```python
from build123d import *

# Parameters (mm, degrees)
SKETCH1_R               = 19.05
BOSS_EXTRUDE1_DEPTH     = 5.08
SKETCH4_R               = 9.398
BOSS_EXTRUDE2_DEPTH     = 7.112
SKETCH5_R               = 2.921
CUT_EXTRUDE1_DEPTH      = 28.863695807
CUT_EXTRUDE1_DEPTH_BACK = 3.429
SKETCH6_R               = 1.4605
SKETCH6_R_2             = 1.73706236
CUT_EXTRUDE2_DEPTH      = 28.863695807
CUT_EXTRUDE2_DEPTH_BACK = 28.863695807
CUT_EXTRUDE5_DEPTH      = 3.175
SKETCH10_R              = 1.5875
CUT_EXTRUDE6_DEPTH      = 7.62


with BuildPart() as part:
    # Sketch1 → Boss-Extrude1 (new body)
    with BuildSketch(Plane(origin=(0, 0, 0), x_dir=(1, 0, 0), z_dir=(0, 1, 0))):
        with Locations(Location((0, 0, 0), (0, 0, 270))):
            Circle(SKETCH1_R)
    extrude(amount=BOSS_EXTRUDE1_DEPTH)

    # Sketch4 → Boss-Extrude2 (add)
    with BuildSketch(Plane(origin=(0, 5.08, 0), x_dir=(1, 0, 0), z_dir=(0, 1, 0))):
        with Locations(Location((0, 0, 0), (0, 0, 270))):
            Circle(SKETCH4_R)
    extrude(amount=BOSS_EXTRUDE2_DEPTH)

    # Sketch5 → Cut-Extrude1 (cut, two sides)
    with BuildSketch(Plane(origin=(0, 5.08, 0), x_dir=(1, 0, 0), z_dir=(0, 1, 0))) as cut_extrude1_sk:
        with Locations(Location((-11.43, 0, 0), (0, 0, 40.395058429))):
            Circle(SKETCH5_R)
        with Locations(Location((11.43, 0, 0), (0, 0, 139.604941571))):
            Circle(SKETCH5_R)
    extrude(amount=CUT_EXTRUDE1_DEPTH, mode=Mode.SUBTRACT)
    extrude(cut_extrude1_sk.sketch, amount=-CUT_EXTRUDE1_DEPTH_BACK, mode=Mode.SUBTRACT)

    # Sketch6 → Cut-Extrude2 (cut, two sides)
    with BuildSketch(Plane(origin=(0, 5.08, 0), x_dir=(1, 0, 0), z_dir=(0, 1, 0))) as cut_extrude2_sk:
        with Locations(Location((-11.43, 0, 0), (0, 0, 270))):
            Circle(SKETCH6_R)
        with Locations(Location((11.43, 0, 0), (0, 0, 270))):
            Circle(SKETCH6_R_2)
    extrude(amount=CUT_EXTRUDE2_DEPTH, mode=Mode.SUBTRACT)
    extrude(cut_extrude2_sk.sketch, amount=-CUT_EXTRUDE2_DEPTH_BACK, mode=Mode.SUBTRACT)

    # Sketch9 → Cut-Extrude5 (cut)
    with BuildSketch(Plane(origin=(0, 12.192, 0), x_dir=(1, 0, 0), z_dir=(0, 1, 0))):
        Polygon((3.299556788, 5.08), (1.649778394, 7.9375), (-1.649778394, 7.9375), (-3.299556788, 5.08), (-1.649778394, 2.2225), (1.649778394, 2.2225), align=None)
        Polygon((3.299556788, -5.08), (1.649778394, -2.2225), (-1.649778394, -2.2225), (-3.299556788, -5.08), (-1.649778394, -7.9375), (1.649778394, -7.9375), align=None)
    extrude(amount=-CUT_EXTRUDE5_DEPTH, mode=Mode.SUBTRACT)

    # Sketch10 → Cut-Extrude6 (cut)
    with BuildSketch(Plane(origin=(0, 12.192, 0), x_dir=(1, 0, 0), z_dir=(0, 1, 0))):
        with Locations(Location((0, 5.08, 0), (0, 0, 270))):
            Circle(SKETCH10_R)
        with Locations(Location((0, -5.08, 0), (0, 0, 270))):
            Circle(SKETCH10_R)
    extrude(amount=-CUT_EXTRUDE6_DEPTH, mode=Mode.SUBTRACT)


solid = part.part
```
Design review of the part built by this model. Coordinates are the model's own, in mm. A direction names the side the tool comes from. Give positions to 0.01 mm unless a question says otherwise; leave off trailing zeros. Write each loop counter-clockwise with the first axis right and the second up, starting at its lowest first coordinate (ties: lowest second). Pieces come first, ordered by that corner, then holes. Notation, with made-up numbers: (19, 71.25) - (74, 71.25) arc R21 cw to (74, 108.25) - close; hole circle Ø5 at (16, -28). An arc over 180 degrees is marked (long way). Return JSON: item names as keys, results as strings. Group by question number.
(1) To check wall thickness, follow probe 1 along X at (y, z) = (5, 0); probe 2 along Z at (x, y) = (-1, 5); probe 3 along Y at (x, z) = (-1.5, -4). State the ranges of each line that lie inside material, in increasing order.
(2) Insertion check: pin 1 (3.5 mm diameter, centred on x = -0.5, y = 10.5, fed in from +Z); pin 2 (3.5 mm diameter, centred on x = 0, z = 5.08, fed in from +Y); pin 3 (5 mm diameter, centred on y = 1.5, z = -0.5, fed in from +X). Each pin has a flat end and moves straight along its axis. Give the tip position at first contact, or say it passes through.
(3) We need section C-C, the plane x = 11.43. Give the boundary of the cut face in (y, z).
(4) Machinability: for faces 1 (the cylindrical face through (0.477, 6.826, 6.594)), 2 (the cylindrical face through (-11.59, 2.5, -15.12)), which of the approach directions +Z, -Z, +X, -X, +Y, -Y give a long, thin tool a straight path to every point of the face, cutting with its end or side? Answer none if there is none.
(5) We need section D-D, the plane x = 0. Give the boundary of the cut face in (y, z), then the cut area to 3 significant figures.
(6) Mouldability with a two-part tool opening along X and no side actions: class faces 3 (the cylindrical face through (-12.856, 0.837, -0.317)), 4 (the flat face through (0, 0, 0)), 5 (the cylindrical face through (0.18, 8.586, -9.396)) as +X half, -X half, draft (parallel to the pull), parting line (faces both ways), or undercut.
(7) We need section A-A, the plane z = 0. Give the boundary of the cut face in (x, y).
(8) We need section B-B, the plane y = 10.75. Give the boundary of the cut face in (x, z).
Reported:
{
 "1": {"probe 1": "x = -19.05 to -14.35, -8.51 to 8.51, 14.35 to 19.05", "probe 2": "z = -19.02 to -6.31, -3.85 to 3.85, 6.31 to 19.02", "probe 3": "y = 0 to 9.02"},
 "2": {"pin 1": "stops at z = 9.4", "pin 2": "stops at y = 9.02", "pin 3": "stops at x = 19.05"},
 "3": {"outline": "(0, -15.24) - (5.08, -15.24) - (5.08, -2.92) - (1.65, -2.92) - (1.65, -1.74) - (0, -1.74) - close; (0, 1.74) - (1.65, 1.74) - (1.65, 2.92) - (5.08, 2.92) - (5.08, 15.24) - (0, 15.24) - close"},
 "4": {"face 1": "+Y", "face 2": "+Y, -Y"},
 "5": {"outline": "(0, -19.05) - (5.08, -19.05) - (5.08, -9.4) - (12.19, -9.4) - (12.19, -7.94) - (9.02, -7.94) - (9.02, -6.67) - (4.57, -6.67) - (4.57, -3.49) - (9.02, -3.49) - (9.02, -2.22) - (12.19, -2.22) - (12.19, 2.22) - (9.02, 2.22) - (9.02, 3.49) - (4.57, 3.49) - (4.57, 6.67) - (9.02, 6.67) - (9.02, 7.94) - (12.19, 7.94) - (12.19, 9.4) - (5.08, 9.4) - (5.08, 19.05) - (0, 19.05) - close", "area": "263 mm2"},
 "6": {"face 3": "undercut", "face 4": "draft", "face 5": "parting line"},
 "7": {"outline": "(-19.05, 0) - (-12.89, 0) - (-12.89, 1.65) - (-14.35, 1.65) - (-14.35, 5.08) - (-19.05, 5.08) - close; (-9.97, 0) - (9.69, 0) - (9.69, 1.65) - (8.51, 1.65) - (8.51, 12.19) - (-8.51, 12.19) - (-8.51, 1.65) - (-9.97, 1.65) - close; (13.17, 0) - (19.05, 0) - (19.05, 5.08) - (14.35, 5.08) - (14.35, 1.65) - (13.17, 1.65) - close"},
 "8": {"outline": "(-9.21, -1.89) arc R9.4 ccw to (9.21, -1.89) arc R2.92 cw to (9.21, 1.89) arc R9.4 ccw to (-9.21, 1.89) arc R2.92 cw to start; hole (-3.3, -5.08) - (-1.65, -7.94) - (1.65, -7.94) - (3.3, -5.08) - (1.65, -2.22) - (-1.65, -2.22) - close; hole (-3.3, 5.08) - (-1.65, 2.22) - (1.65, 2.22) - (3.3, 5.08) - (1.65, 7.94) - (-1.65, 7.94) - close"}
}
